```python
from build123d import *

# Parameters (mm, degrees)
F0_R     = 7
F0_R_2   = 4
F1_DEPTH = 3
F2_R     = 5
F2_R_2   = 4
F3_DEPTH = 3
F5_DEPTH = 6


with BuildPart() as f1:
    # F0 (on Top) → F1 (new body)
    with BuildSketch(Plane.XY):
        Circle(F0_R)
        Circle(F0_R_2, mode=Mode.SUBTRACT)
    extrude(amount=F1_DEPTH)

    # F2 (on face) → F3 (join)
    with BuildSketch(Plane.XY.offset(3)):
        Circle(F2_R)
        Circle(F2_R_2, mode=Mode.SUBTRACT)
    extrude(amount=F3_DEPTH)

    # F4 (on Top) → F5 (cut, through all)
    with BuildSketch(Plane.XY):
        with BuildLine():
            Line((0.4, 5), (4.8989794856, 5))
            ThreePointArc((4.8989794856, 5), (0, 7), (-4.8989794856, 5))
            Line((-4.8989794856, 5), (-0.4, 5))
            Line((-0.4, 5), (0, 5))
            Line((0, 5), (0.4, 5))
        make_face()
        Polygon((0.4, 3.376792185), (0.4, 5), (0, 5), (-0.4, 5), (-0.4, 3.376792185), align=None)
    extrude(amount=F5_DEPTH, mode=Mode.SUBTRACT)


solid = f1.part
```
Can you work these out from the model? Positions are in its coordinate system, mm. A direction names the side the tool comes from. Coordinates: 2 decimals unless noted, no trailing zeros. Loops run counter-clockwise (first coordinate to the right, second up) from the corner with the lowest first, then second, coordinate; pieces in that order, holes last. Notation, with made-up numbers: (63.5, -19) -> (92.5, -19) arc R20 cw to (92.5, 15) -> close; hole circle Ø4 at (-19, 89). An arc over 180 degrees is marked (long way). Answer as a JSON object with one key per item and string values.
1) If I drill on line 1 (X direction, y = 0, z = 1.6); line 2 (X direction, y = 0, z = 5.75); line 3 (Z direction, x = -5.5, y = 2), over which ranges is the centre line in solid material (lowest first)?
Results:
{"line 1": "x = -7 to -4, 4 to 7", "line 2": "x = -5 to -4, 4 to 5", "line 3": "z = 0 to 3"}
2) Thinking about a two-plate mould opening in Y: for faces 1 (the face through (0, -4, 3)), 2 (the face through (0, -5, 4)), 3 (the face through (-2, -5, 3)), 4 (the face through (3, 5, 1)), which applies, pulls with the +Y half, pulls with the -Y half, needs draft (parallel to the pull), parting line crosses it, or undercut?
Results:
{"face 1": "undercut", "face 2": "parting line crosses it", "face 3": "needs draft", "face 4": "pulls with the +Y half"}
3) For P1, Ø1.1, axis at y = 4.5, z = 2, coming from the +X side; P2, Ø0.5, axis at y = 4.5, z = 4.5, coming from the -X side; P3, Ø1.5, axis at y = 3.5, z = 3.5, coming from the -X side, each with a flat end and sliding along its axis, tell me the tip position at first contact or that it passes through.
Results:
{"P1": "stops at x = 5.78", "P2": "stops at x = -2.63", "P3": "stops at x = -6.35"}
4) Imagine slicing it at A-A (y = 0). Please give me the cut outline in (x, z), then the cut area to 3 significant figures.
Results:
{"outline": "(-7, 0) -> (-4, 0) -> (-4, 6) -> (-5, 6) -> (-5, 3) -> (-7, 3) -> close; (4, 0) -> (7, 0) -> (7, 3) -> (5, 3) -> (5, 6) -> (4, 6) -> close", "area": "24.0 mm^2"}
5) Imagine slicing it at D-D (x = 0). Please give me the cut outline in (y, z), then the cut area to 3 significant figures.
Results:
{"outline": "(-7, 0) -> (-4, 0) -> (-4, 6) -> (-5, 6) -> (-5, 3) -> (-7, 3) -> close", "area": "12.0 mm^2"}
6) Imagine slicing it at B-B (x = -1.5). Please give me the cut outline in (y, z).
Results:
{"outline": "(-6.84, 0) -> (-3.71, 0) -> (-3.71, 6) -> (-4.77, 6) -> (-4.77, 3) -> (-6.84, 3) -> close; (3.71, 0) -> (5, 0) -> (5, 3) -> (4.77, 3) -> (4.77, 6) -> (3.71, 6) -> close"}
7) Imagine slicing it at C-C (z = 1.1). Please give me the cut outline in (x, y).
Results:
{"outline": "(-4.9, 5) arc R7 ccw (long way) to (4.9, 5) -> (0.4, 5) -> (0.4, 3.98) arc R4 cw (long way) to (-0.4, 3.98) -> (-0.4, 5) -> close"}
8) For faces 5 (the face through (-2, 4, 6)), 6 (the face through (-0.4, 4.5, 3)), which set-ups out of +Z, -Z, +X, -X, +Y, -Y let a thin tool reach every point of the face, with its end or its side?
Results:
{"face 5": "+Z, +X, -X, +Y, -Y", "face 6": "+Z, -Z, +Y"}
